The listing builds one solid part. Answer for the finished solid, in the listing's coordinates (mm). A direction names the side the tool comes from. Give positions to 0.01 mm unless a question says otherwise; leave off trailing zeros. Order: outer loops, then holes, each group sorted by start corner. A loop starts at its lowest first (then second) coordinate and runs counter-clockwise, first axis right, second up. Notation, with made-up numbers: (38, 67.5) - (46, 67.5) arc R32 cw to (46, 102.5) - close; hole circle Ø2 at (26.5, 14.25). An arc over 180 degrees is marked (long way). Use a Markdown table: item, result. Add a question column.
1) The mould has two halves that part along Z. Classify faces 4 (the face through (0, 5.5, 1)), 5 (the face through (0, 4, 4)), 6 (the face through (0, 0, 26.5)), 7 (the face through (0, -6, 0)): released by +Z, released by -Z, zero draft, split by the parting line, or undercut.
2) Flat-ended cylindrical pins translate along their axes: pin 1 (2.5 mm diameter, centred on x = 0, y = 0, fed in from -Z); pin 2 (5 mm diameter, centred on x = 4, z = 16, fed in from -Y); pin 3 (5 mm diameter, centred on x = 1, y = 1, fed in from -Z). Find the tip coordinate at first contact, or state that the pin passes through.
3) Find section D-D, the plane x = 3.5. Determine the outline of the cut face in (y, z).
4) For faces 1 (the face through (0, -5.5, 1)), 2 (the face through (-5.5, 0, 39)), 3 (the face through (4, 2, 6)), determine the directions among +Z, -Z, +X, -X, +Y, -Y from which every point of the face is accessible in a straight line to the end or side of a thin tool.
5) Find section B-B, the plane z = 11.5. Determine the outline of the cut face in (x, y), plus the area to 3 significant figures.
6) Find section C-C, the plane y = 4.25. Determine the outline of the cut face in (x, z).
7) Find section A-A, the plane x = 0. State how many separate pieces and enclosed holes the cut face has, plus the area to 3 significant figures.
8) Straight lines are drawn through the part: line 1 (Z direction, x = -3.25, y = 7.5); line 2 (Z direction, x = -2.25, y = 3.25); line 3 (Y direction, x = 0, z = 9.55). For each, find the intervals that lie inside material, in ascending order.
from build123d import *

# Parameters (mm, degrees)
SKETCH_R        = 9
PAD_DEPTH       = 40
SKETCH001_W     = 11
SKETCH001_H     = 11
POCKET_DEPTH    = 1.5
SKETCH002_W     = 11
SKETCH002_H     = 11
POCKET001_DEPTH = 1.5
SKETCH003_R     = 2.25
POCKET002_DEPTH = 12
SKETCH004_R     = 2.25
POCKET003_DEPTH = 12
SKETCH005_W     = 8
SKETCH005_H     = 4
POCKET004_DEPTH = 20


with BuildPart() as part:
    # Sketch → Pad (new body)
    with BuildSketch(Plane.XY):
        Circle(SKETCH_R)
    extrude(amount=PAD_DEPTH)

    # Sketch001 (on Face3 of Pad) → Pocket (cut)
    with BuildSketch(Plane.XY.offset(40)):
        Rectangle(SKETCH001_W, SKETCH001_H)
    extrude(amount=-POCKET_DEPTH, mode=Mode.SUBTRACT)

    # Sketch002 (on Face2 of Pocket) → Pocket001 (cut)
    with BuildSketch(Plane(origin=(0, 0, 0), x_dir=(1, 0, 0), z_dir=(0, 0, -1))):
        Rectangle(SKETCH002_W, SKETCH002_H)
    extrude(amount=-POCKET001_DEPTH, mode=Mode.SUBTRACT)

    # Sketch003 (on Face12 of Pocket001) → Pocket002 (cut)
    with BuildSketch(Plane(origin=(0, 0, 1.5), x_dir=(1, 0, 0), z_dir=(0, 0, -1))):
        Circle(SKETCH003_R)
    extrude(amount=-POCKET002_DEPTH, mode=Mode.SUBTRACT)

    # Sketch004 (on Face13 of Pocket001) → Pocket003 (cut)
    with BuildSketch(Plane.XY.offset(38.5)):
        Circle(SKETCH004_R)
    extrude(amount=-POCKET003_DEPTH, mode=Mode.SUBTRACT)

    # Sketch005 → Pocket004 (cut)
    with BuildSketch(Plane.XZ.offset(4.5)):
        with Locations((0, 6)):
            Rectangle(SKETCH005_W, SKETCH005_H)
        with Locations((0, 34)):
            Rectangle(SKETCH005_W, SKETCH005_H)
    extrude(amount=-POCKET004_DEPTH, mode=Mode.SUBTRACT)


solid = part.part
The answers:
| question | item | result |
|---|---|---|
| 1 | face 4 | zero draft |
| 1 | face 5 | undercut |
| 1 | face 6 | released by +Z |
| 1 | face 7 | released by -Z |
| 2 | pin 1 | z = 13.5 |
| 2 | pin 2 | y = -8.87 |
| 2 | pin 3 | z = 1.5 |
| 3 | outline | (-8.29, 0) - (-5.5, 0) - (-5.5, 1.5) - (5.5, 1.5) - (5.5, 0) - (8.29, 0) - (8.29, 4) - (-4.5, 4) - (-4.5, 8) - (8.29, 8) - (8.29, 32) - (-4.5, 32) - (-4.5, 36) - (8.29, 36) - (8.29, 40) - (5.5, 40) - (5.5, 38.5) - (-5.5, 38.5) - (-5.5, 40) - (-8.29, 40) - close |
| 4 | face 1 | -Z |
| 4 | face 2 | +Z |
| 4 | face 3 | +Y |
| 5 | outline | circle Ø18 at (0, 0); hole circle Ø4.5 at (0, 0) |
| 5 | area | 239 mm2 |
| 6 | outline | (-7.93, 0) - (-5.5, 0) - (-5.5, 1.5) - (5.5, 1.5) - (5.5, 0) - (7.93, 0) - (7.93, 40) - (5.5, 40) - (5.5, 38.5) - (-5.5, 38.5) - (-5.5, 40) - (-7.93, 40) - close; hole (-4, 4) - (4, 4) - (4, 8) - (-4, 8) - close; hole (-4, 32) - (4, 32) - (4, 36) - (-4, 36) - close |
| 7 | separate pieces | 3 |
| 7 | enclosed holes | 0 |
| 7 | area | 507 mm2 |
| 8 | line 1 | 0 to 4, 8 to 32, 36 to 40 |
| 8 | line 2 | 1.5 to 4, 8 to 32, 36 to 38.5 |
| 8 | line 3 | -9 to -2.25, 2.25 to 9 |
